from build123d import *

# Parameters (mm, degrees)
CYLINDER002_R     = 0.6
CYLINDER002_DEPTH = 100
ARRAY003_X_COUNT  = 8
ARRAY003_X_PITCH  = 20
BOX009_W          = 15
BOX009_H          = 25.76
BOX009_DEPTH      = 10
BOX010_W          = 30
BOX010_H          = 25.76
BOX010_DEPTH      = 10
BOX011_W          = 18
BOX011_H          = 25.76
BOX011_DEPTH      = 10
CYLINDER004_R     = 4
CYLINDER004_DEPTH = 10
BOX012_W          = 2
BOX012_H          = 8.76
BOX012_DEPTH      = 21.3
BOX005_W          = 166
BOX005_H          = 17.76
BOX005_DEPTH      = 6
BOX006_W          = 170
BOX006_H          = 25.76
BOX006_DEPTH      = 2
BOX008_W          = 2
BOX008_H          = 20.76
BOX008_DEPTH      = 25.8
BOX007_W          = 2
BOX007_H          = 20.76
BOX007_DEPTH      = 22.2
BOX004_W          = 170
BOX004_H          = 20.96
BOX004_DEPTH      = 6


with BuildPart() as array003:
    # Cylinder002 → Cylinder002 (new body)
    with BuildSketch(Plane(origin=(18.5, -32.5, 23), x_dir=(1, 0, 0), z_dir=(0, 1, 0))):
        Circle(CYLINDER002_R)
    extrude(amount=CYLINDER002_DEPTH)

    # Array003 X: Array003 ×8


with BuildPart() as array003_1:
    add(array003.part)
    with Locations(*[(i * ARRAY003_X_PITCH, 0, 0) for i in range(1, ARRAY003_X_COUNT)]):
        add(array003.part)


with BuildPart() as cube009:
    # Box009 → Box009 (new body)
    with BuildSketch(Plane.XY.offset(16)):
        with Locations((7.5, 12.88)):
            Rectangle(BOX009_W, BOX009_H)
    extrude(amount=BOX009_DEPTH)


with BuildPart() as cube010:
    # Box010 → Box010 (new body)
    with BuildSketch(Plane(origin=(64, 0, 16), x_dir=(1, 0, 0), z_dir=(0, 0, 1))):
        with Locations((15, 12.88)):
            Rectangle(BOX010_W, BOX010_H)
    extrude(amount=BOX010_DEPTH)


with BuildPart() as cube011:
    # Box011 → Box011 (new body)
    with BuildSketch(Plane(origin=(148, 0, 16), x_dir=(1, 0, 0), z_dir=(0, 0, 1))):
        with Locations((9, 12.88)):
            Rectangle(BOX011_W, BOX011_H)
    extrude(amount=BOX011_DEPTH)


with BuildPart() as cylinder004:
    # Cylinder004 → Cylinder004 (new body)
    with BuildSketch(Plane(origin=(51.5, 12.88, 20), x_dir=(1, 0, 0), z_dir=(0, 0, 1))):
        Circle(CYLINDER004_R)
    extrude(amount=CYLINDER004_DEPTH)


with BuildPart() as cube012:
    # Box012 → Box012 (new body)
    with BuildSketch(Plane(origin=(166, 8.5, 0), x_dir=(1, 0, 0), z_dir=(0, 0, 1))):
        with Locations((1, 4.38)):
            Rectangle(BOX012_W, BOX012_H)
    extrude(amount=BOX012_DEPTH)


with BuildPart() as cut_out_fusion:
    # Box005 → Box005 (new body)
    with BuildSketch(Plane(origin=(0, 4, 19), x_dir=(1, 0, 0), z_dir=(0, 0, 1))):
        with Locations((83, 8.88)):
            Rectangle(BOX005_W, BOX005_H)
    extrude(amount=BOX005_DEPTH)

    # Fusion002: union Array003, Cube009, Cube010, Cube011, Cylinder004, Cube012
    add(array003_1.part)
    add(cube009.part)
    add(cube010.part)
    add(cube011.part)
    add(cylinder004.part)
    add(cube012.part)


with BuildPart() as cube006:
    # Box006 → Box006 (new body)
    with BuildSketch(Plane.XY.offset(26.4)):
        with Locations((85, 12.88)):
            Rectangle(BOX006_W, BOX006_H)
    extrude(amount=BOX006_DEPTH)


with BuildPart() as cube008:
    # Box008 → Box008 (new body)
    with BuildSketch(Plane(origin=(168, 2.5, 2.5), x_dir=(1, 0, 0), z_dir=(0, 0, 1))):
        with Locations((1, 10.38)):
            Rectangle(BOX008_W, BOX008_H)
    extrude(amount=BOX008_DEPTH)


with BuildPart() as cube007:
    # Box007 → Box007 (new body)
    with BuildSketch(Plane(origin=(166, 2.5, 2.5), x_dir=(1, 0, 0), z_dir=(0, 0, 1))):
        with Locations((1, 10.38)):
            Rectangle(BOX007_W, BOX007_H)
    extrude(amount=BOX007_DEPTH)


with BuildPart() as lid_cut:
    # Box004 → Box004 (new body)
    with BuildSketch(Plane(origin=(0, 2.4, 21), x_dir=(1, 0, 0), z_dir=(0, 0, 1))):
        with Locations((85, 10.48)):
            Rectangle(BOX004_W, BOX004_H)
    extrude(amount=BOX004_DEPTH)

    # Fusion001: union Cube006, Cube008, Cube007
    add(cube006.part)
    add(cube008.part)
    add(cube007.part)

    # Cut002: cut cut out fusion
    add(cut_out_fusion.part, mode=Mode.SUBTRACT)


solid = lid_cut.part
Verification items for the finished model (mm, model axes). A direction names the side the tool comes from. Round coordinates to 2 decimals unless told otherwise and drop trailing zeros. Loops run counter-clockwise (first coordinate to the right, second up) from the corner with the lowest first, then second, coordinate; pieces in that order, holes last. Notation, with made-up numbers: (-37.75, 76.5) - (-32.75, 76.5) arc R9 ccw to (-32.75, 86.5) - close; hole circle Ø10 at (65.25, 4.25). An arc over 180 degrees is marked (long way). Write item = value, one per line.
Q1. Material ranges on L1, parallel to Z at x = 38.5, y = 3.45; L2, parallel to Y at x = 122, z = 24.5; L3, parallel to X at y = 13, z = 26.5, recorded low to high.
Here are the results:
L1 = 21 to 22.4, 23.6 to 28.4
L2 = 2.4 to 4, 21.76 to 23.36
L3 = 0 to 47.5, 55.5 to 170
Q2. Sectioned sample at D-D on x = 33. Record the boundary of the cut face in (y, z), plus the area to 3 significant figures.
Here are the results:
outline = (0, 26.4) - (2.4, 26.4) - (2.4, 21) - (4, 21) - (4, 25) - (21.76, 25) - (21.76, 21) - (23.36, 21) - (23.36, 26.4) - (25.76, 26.4) - (25.76, 28.4) - (0, 28.4) - close
area = 93.7 mm^2
Q3. Depth check by flat-ended pin: pin 1 (6.5 mm diameter, centred on x = 51.5, y = 12.88, fed in from -Z); pin 2 (1 mm diameter, centred on x = 167, z = 14, fed in from -Y); pin 3 (3 mm diameter, centred on x = 151.5, y = 3.5, fed in from -Z); pin 4 (2.5 mm diameter, centred on y = 14.5, z = 23.5, fed in from -X). Enter the tip coordinate at first touch or a pass-through.
Here are the results:
pin_1 = through
pin_2 = 2.5
pin_3 = 26
pin_4 = 166
Q4. Sectioned sample at C-C on y = 10.75. Record the boundary of the cut face in (x, z).
Here are the results:
outline = (0, 26) - (15, 26) - (15, 25) - (48.11, 25) - (48.11, 28.4) - (0, 28.4) - close; (54.89, 25) - (64, 25) - (64, 26) - (94, 26) - (94, 25) - (148, 25) - (148, 26) - (166, 26) - (166, 21.3) - (168, 21.3) - (168, 2.5) - (170, 2.5) - (170, 28.4) - (54.89, 28.4) - close
Q5. Tool access check on faces 1 (the flat face through (7, 13, 26)), 2 (the flat face through (103, 23.36, 24)), 3 (the flat face through (79, 13, 26)), 4 (the flat face through (168.4, 13, 2.5)), 5 (the flat face through (39.2, 4, 23.4)). Record the directions out of +Z, -Z, +X, -X, +Y, -Y that give a thin tool (end or side, any length) a straight path to the whole face; none if there is none.
Here are the results:
face_1 = -Z, -X, +Y, -Y
face_2 = -Z, +X, -X, +Y
face_3 = -Z, +Y, -Y
face_4 = -Z, +X, -X, +Y, -Y
face_5 = -Z, -X
Q6. Sectioned sample at A-A on z = 6.5. Record the boundary of the cut face in (x, y), plus the area to 3 significant figures.
Here are the results:
outline = (166, 2.5) - (170, 2.5) - (170, 23.26) - (166, 23.26) - (166, 17.26) - (168, 17.26) - (168, 8.5) - (166, 8.5) - close
area = 65.5 mm^2
Q7. Sectioned sample at B-B on x = 71. Record the boundary of the cut face in (y, z).
Here are the results:
outline = (0, 26.4) - (2.4, 26.4) - (2.4, 26) - (23.36, 26) - (23.36, 26.4) - (25.76, 26.4) - (25.76, 28.4) - (0, 28.4) - close
Q8. Mould release check, pull along X, two halves, no side actions. Record for faces 6 (the flat face through (170, 13, 15)), 7 (the flat face through (157, 13, 26)), 8 (the flat face through (168, 13, 12)), 9 (the flat face through (168, 23.26, 12)): +X half, -X half, draft (parallel to the pull), parting line (faces both ways), or undercut.
Here are the results:
face_6 = +X half
face_7 = undercut
face_8 = -X half
face_9 = draft
